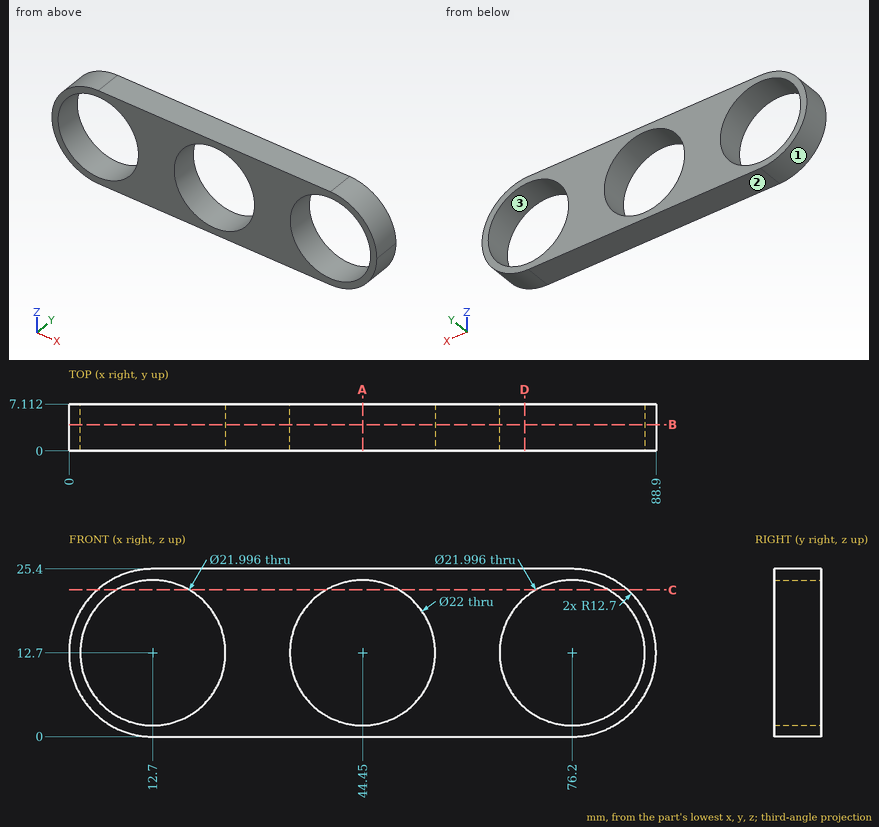
Input: dimensioned drawing with shaded views. Units: mm. Origin: part minimum x, y, z. Give positions to 0.01 mm unless a question says otherwise; leave off trailing zeros. Write each loop counter-clockwise with the first axis right and the second up, starting at its lowest first coordinate (ties: lowest second). Pieces come first, ordered by that corner, then holes.
1. Pin query (flat end, axial travel): P1, Ø2, axis at y = 2.5, z = 11.5, coming from the +X side. Return the tip coordinate at first contact, or that it passes through.
2. Draft query along Z for the marked faces 1, 2 and 3. Return one class per face: released by +Z, released by -Z, zero draft, split by the parting line, or undercut.
3. Section query C-C, the plane z = 22.25. Return loops of the section in (x, y) (1 decimal), then the cut area to 3 significant figures.
4. Section query D-D, the plane x = 69. Return loops of the section in (y, z), then the cut area to 3 significant figures.
5. Line query: probe 1 along X at (y, z) = (3.5, 5.75) (1 decimal); probe 2 along X at (y, z) = (3.5, 22.5) (1 decimal); probe 3 along Z at (x, y) = (76.2, 5.25). Output: solid intervals per line, ascending.
6. Section query A-A, the plane x = 44.45. Return loops of the section in (y, z).
7. Section query B-B, the plane y = 4. Return loops of the section in (x, z).
Computed:
1. P1: stops at x = 88.9
2. face 1: split by the parting line
2. face 2: released by -Z
2. face 3: undercut
3. outline: (4.3, 0) - (7.2, 0) - (7.2, 7.1) - (4.3, 7.1) - close; (18.2, 0) - (39, 0) - (39, 7.1) - (18.2, 7.1) - close; (49.9, 0) - (70.7, 0) - (70.7, 7.1) - (49.9, 7.1) - close; (81.7, 0) - (84.6, 0) - (84.6, 7.1) - (81.7, 7.1) - close
3. area: 338 mm2
4. outline: (0, 0) - (7.11, 0) - (7.11, 4.39) - (0, 4.39) - close; (0, 21.01) - (7.11, 21.01) - (7.11, 25.4) - (0, 25.4) - close
4. area: 62.4 mm2
5. probe 1: x = 2.1 to 4.2, 21.2 to 35.9, 53 to 67.7, 84.7 to 86.8
5. probe 2: x = 4.6 to 7.7, 17.7 to 39.5, 49.4 to 71.2, 81.2 to 84.3
5. probe 3: z = 0 to 1.7, 23.7 to 25.4
6. outline: (0, 0) - (7.11, 0) - (7.11, 1.7) - (0, 1.7) - close; (0, 23.7) - (7.11, 23.7) - (7.11, 25.4) - (0, 25.4) - close
7. outline: (12.7, 0) - (76.2, 0) arc R12.7 ccw to (76.2, 25.4) - (12.7, 25.4) arc R12.7 ccw to start; hole circle Ø22 at (12.7, 12.7); hole circle Ø22 at (44.45, 12.7); hole circle Ø22 at (76.2, 12.7)
